For this review, take the finished solid that the model builds, in its own axes (mm). Round coordinates to 2 decimals unless told otherwise and drop trailing zeros. Order: outer loops, then holes, each group sorted by start corner. A loop starts at its lowest first (then second) coordinate and runs counter-clockwise, first axis right, second up. Notation, with made-up numbers: M -19,59 L 28,59 A29 ccw 28,86 Z; hole C 25,-5.75 d1. An arc over 180 degrees is marked long. Use a Markdown table: item, result.
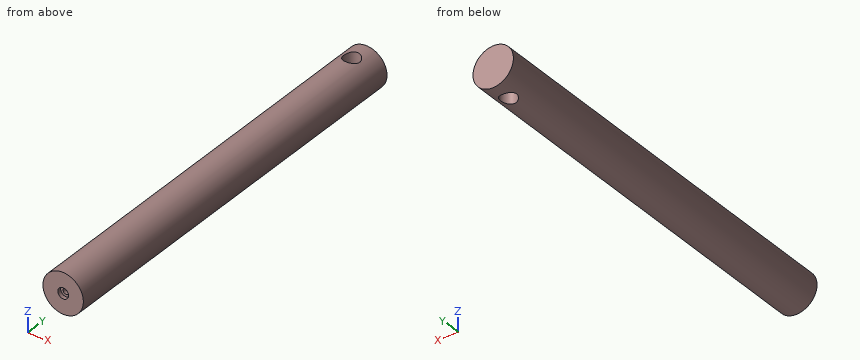
from build123d import *

# Parameters (mm, degrees)
SKETCH1_R               = 15
BOSS_EXTRUDE1_DEPTH     = 300
SKETCH2_R               = 6
CUT_EXTRUDE1_DEPTH      = 16
CUT_EXTRUDE1_DEPTH_BACK = 16
SKETCH3_R               = 4
CUT_EXTRUDE2_DEPTH      = 2.85
SKETCH4_R               = 2.25
CUT_EXTRUDE3_DEPTH      = 2.5


with BuildPart() as part:
    # Sketch1 → Boss-Extrude1 (new body)
    with BuildSketch(Plane(origin=(0, 0, 0), x_dir=(1, 0, 0), z_dir=(0, 1, 0))):
        Circle(SKETCH1_R)
    extrude(amount=BOSS_EXTRUDE1_DEPTH)

    # Sketch2 → Cut-Extrude1 (cut, two sides)
    with BuildSketch(Plane.XY) as cut_extrude1_sk:
        with Locations((0, 285)):
            Circle(SKETCH2_R)
    extrude(amount=CUT_EXTRUDE1_DEPTH, mode=Mode.SUBTRACT)
    extrude(cut_extrude1_sk.sketch, amount=-CUT_EXTRUDE1_DEPTH_BACK, mode=Mode.SUBTRACT)

    # Sketch3 → Cut-Extrude2 (cut)
    with BuildSketch(Plane.XZ):
        Circle(SKETCH3_R)
    extrude(amount=-CUT_EXTRUDE2_DEPTH, mode=Mode.SUBTRACT)

    # Sketch4 → Cut-Extrude3 (cut)
    with BuildSketch(Plane.XZ.offset(-2.85)):
        Circle(SKETCH4_R)
    extrude(amount=-CUT_EXTRUDE3_DEPTH, mode=Mode.SUBTRACT)


solid = part.part
Q1. Add section D-D (z = -6.5). Write out the cut boundary in (x, y).
Determined:
| item | result |
|---|---|
| outline | M -13.52,0 L 13.52,0 L 13.52,300 L -13.52,300 Z; hole C 0,285 d12 |
Q2. Add section A-A (z = 9). Write out the cut boundary in (x, y), then the cut area to 3 significant figures.
Determined:
| item | result |
|---|---|
| outline | M -12,0 L 12,0 L 12,300 L -12,300 Z; hole C 0,285 d12 |
| area | 7,090 mm^2 |
Q3. Add section B-B (y = 178.5). Write out the cut boundary in (x, z), then the cut area to 3 significant figures.
Determined:
| item | result |
|---|---|
| outline | C 0,0 d30 |
| area | 707 mm^2 |
Q4. Wall thickness on line 1 along Z through (x, y) = (0, 2.1); line 2 along Y through (x, z) = (0, -8); line 3 along Z through (x, y) = (1, 196.5): over which ranges is each line inside the solid? List them lowest first. Write a range as [from, to].
Determined:
| item | result |
|---|---|
| line 1 | z = [-15, -4], [4, 15] |
| line 2 | y = [0, 279], [291, 300] |
| line 3 | z = [-14.97, 14.97] |
Q5. Add section C-C (y = 285). Write out the cut boundary in (x, z), then the cut area to 3 significant figures.
Determined:
| item | result |
|---|---|
| outline | M -6,-13.75 L -6,13.75 A15 ccw Z; M 6,-13.75 A15 ccw 6,13.75 Z |
| area | 357 mm^2 |
Q6. Clearance check with flat-ended pins moving along their axes: pin 1 (10 mm diameter, centred on y = 240, z = 6, fed in from -X); pin 2 (5 mm diameter, centred on x = 10.5, y = 54, fed in from +Z); pin 3 (3 mm diameter, centred on y = 131.5, z = -5.5, fed in from -X). State where each tip first meets the part, or that it passes through.
Determined:
| item | result |
|---|---|
| pin 1 | stops at x = -14.97 |
| pin 2 | stops at z = 12.69 |
| pin 3 | stops at x = -14.46 |
